```python
from build123d import *

# Parameters (mm, degrees)
F2_SIZE = 1
F3_R    = 0.5


with BuildPart() as f1:
    # F0 (on Front) → F1 (revolve)
    with BuildSketch(Plane.XZ):
        Polygon((0, 5.08), (0, 2.54), (-3.175, 2.54), (-3.175, 0), (2.54, 0), (2.54, 5.08), align=None)
    revolve(axis=Axis((-24.3718145439, 0, 0), (-1, 0, 0)))

    # F2
    f2_edges = [f1.edges().sort_by_distance(p)[0] for p in [
        (-3.175, 0, -2.54),
    ]]
    chamfer(f2_edges, length=F2_SIZE)

    # F3
    f3_edges = [f1.edges().sort_by_distance(p)[0] for p in [
        (0, 0, -5.08),
        (2.54, 0, -5.08),
    ]]
    fillet(f3_edges, radius=F3_R)


solid = f1.part
```
Verification items for the finished model (mm, model axes). A direction names the side the tool comes from. Coordinates: 2 decimals unless noted, no trailing zeros. Write each loop counter-clockwise with the first axis right and the second up, starting at its lowest first coordinate (ties: lowest second). Pieces come first, ordered by that corner, then holes. Notation, with made-up numbers: M 0,2.25 L 27,2.25 A17 cw 27,31.25 Z; hole C 67,-20 d6. An arc over 180 degrees is marked long. Answer as a JSON object with one key per item and string values. Group by question number.
(1) Cross-section at D-D, the plane x = 1.05. Record the cut outline in (y, z), and give its area (3 significant figures).
(2) Gauge pin test, flat ends, axial feed: pin 1 (2 mm diameter, centred on x = -1.5, z = -1.5, fed in from +Y); pin 2 (2 mm diameter, centred on x = 0, y = -3, fed in from -Z); pin 3 (4 mm diameter, centred on y = -3.5, z = 3.5, fed in from -X). Record the tip position at first contact, or that the pin passes through.
(3) Tool access check on faces 1 (the face through (0, -2, 2)), 2 (the face through (-3.175, 0, 0)). Record the directions out of +Z, -Z, +X, -X, +Y, -Y that give a thin tool (end or side, any length) a straight path to the whole face; none if there is none.
(4) Cross-section at A-A, the plane y = 0. Record the cut outline in (x, z) (3 decimals), and give its area (3 significant figures).
(5) Material ranges on line 1 (X direction, y = -1.25, z = -3.5); line 2 (Z direction, x = 0.15, y = 1.5); line 3 (Y direction, x = 1.75, z = -0.75), recorded low to high.
(6) Cross-section at C-C, the plane x = -1.25. Record the cut outline in (y, z).
Reply:
{
 "1": {"outline": "C 0,0 d10.16", "area": "81.1 mm²"},
 "2": {"pin 1": "y = 2.49", "pin 2": "z = -4.62", "pin 3": "x = 0"},
 "3": {"face 1": "-X", "face 2": "+Z, -Z, -X, +Y, -Y"},
 "4": {"outline": "M -3.175,-1.54 L -2.175,-2.54 L 0,-2.54 L 0,-4.58 A0.5 ccw 0.5,-5.08 L 2.04,-5.08 A0.5 ccw 2.54,-4.58 L 2.54,4.58 A0.5 ccw 2.04,5.08 L 0.5,5.08 A0.5 ccw 0,4.58 L 0,2.54 L -2.175,2.54 L -3.175,1.54 Z", "area": "40.7 mm²"},
 "5": {"line 1": "0 to 2.54", "line 2": "-4.7 to 4.7", "line 3": "-5.02 to 5.02"},
 "6": {"outline": "C 0,0 d5.08"}
}
